Read the model definition and answer for the solid it produces. Units are mm, in the model's axes. Round coordinates to 2 decimals unless told otherwise and drop trailing zeros. Write each loop counter-clockwise with the first axis right and the second up, starting at its lowest first coordinate (ties: lowest second). Pieces come first, ordered by that corner, then holes. Notation, with made-up numbers: (43, -13.75) -> (101, -13.75) arc R30 ccw to (101, 12.25) -> close; hole circle Ø6 at (49.5, 34.25). An arc over 180 degrees is marked (long way). Return JSON: item names as keys, results as strings.
from build123d import *

# Parameters (mm, degrees)
F0_R     = 21
F1_DEPTH = 3
F2_R     = 3.248876
F2_R_2   = 2.201596
F2_R_3   = 3.392524
F2_R_4   = 2.223105
F2_R_5   = 3.218428
F2_R_6   = 2.097756
F3_DEPTH = 25
F4_R     = 3.419132
F5_DEPTH = 25


with BuildPart() as f1:
    # F0 (on Front) → F1 (new body)
    with BuildSketch(Plane.XZ):
        Circle(F0_R)
    extrude(amount=F1_DEPTH)

    # F2 (on Front) → F3 (cut)
    with BuildSketch(Plane.XZ):
        with Locations((0, 28.620865)):
            Circle(F2_R)
        with Locations((0, 28.620865)):
            Circle(F2_R_2, mode=Mode.SUBTRACT)
        with Locations((24.881644, -14.200577)):
            Circle(F2_R_3)
        with Locations((24.881644, -14.200577)):
            Circle(F2_R_4, mode=Mode.SUBTRACT)
        with Locations((-24.80519, -14.200577)):
            Circle(F2_R_5)
        with Locations((-24.80519, -14.200577)):
            Circle(F2_R_6, mode=Mode.SUBTRACT)
    extrude(amount=-F3_DEPTH, mode=Mode.SUBTRACT)

    # F4 (on Front) → F5 (cut)
    with BuildSketch(Plane.XZ):
        with Locations((0, 28.712314)):
            Circle(F4_R)
    extrude(amount=-F5_DEPTH, mode=Mode.SUBTRACT)


solid = f1.part
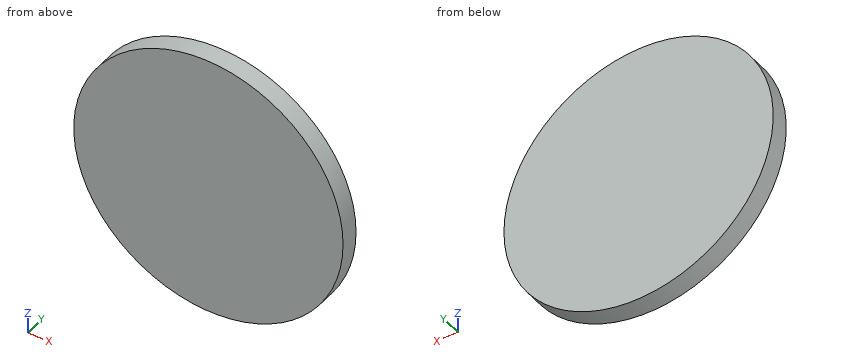
Item 1: Straight lines are drawn through the part: L1, parallel to Z at x = -0.5, y = -0.85; L2, parallel to Z at x = -1.5, y = -0.6; L3, parallel to X at y = -2.05, z = 18. For each, find the intervals that lie inside material, in ascending order. Write a range as [from, to].
Worked answers:
{"L1": "z = [-20.99, 20.99]", "L2": "z = [-20.95, 20.95]", "L3": "x = [-10.82, 10.82]"}
Item 2: Section A-A (y = -2.4) is taken. Give the vertices of the cut face in (x, z).
Worked answers:
{"outline": "circle Ø42 at (0, 0)"}
Item 3: Section C-C (x = -6.5) is taken. Give the vertices of the cut face in (y, z), then the cut area to 3 significant figures.
Worked answers:
{"outline": "(-3, -19.97) -> (0, -19.97) -> (0, 19.97) -> (-3, 19.97) -> close", "area": "120 mm2"}
Item 4: Flat-ended cylindrical pins translate along their axes: pin 1 (1 mm diameter, centred on x = -8.5, y = -2.5, fed in from -Z); pin 2 (1.5 mm diameter, centred on x = 2.5, z = -2.5, fed in from +Y). Find the tip coordinate at first contact, or state that the pin passes through.
Worked answers:
{"pin 1": "stops at z = -19.42", "pin 2": "stops at y = 0"}
Item 5: Section B-B (z = -17) is taken. Give the vertices of the cut face in (x, y).
Worked answers:
{"outline": "(-12.33, -3) -> (12.33, -3) -> (12.33, 0) -> (-12.33, 0) -> close"}
